Input: dimensioned drawing with shaded views. Units: mm. Origin: part minimum x, y, z. A direction names the side the tool comes from. Coordinates: 2 decimals unless noted, no trailing zeros. Loops run counter-clockwise (first coordinate to the right, second up) from the corner with the lowest first, then second, coordinate; pieces in that order, holes last. Notation, with made-up numbers: (11.5, 46) - (35.5, 46) arc R21 cw to (35.5, 63) - close; hole circle Ø8 at (62.25, 54.25). An arc over 180 degrees is marked (long way). Put each result on its own line as item: value. Start each with the question number.
1) Contact query for flat-ended pins moving along their axis: pin 1 Ø8 at (x, y) = (13.5, 17) entering from +Z; pin 2 Ø1 at (y, z) = (32, 7) entering from +X; pin 3 Ø6 at (x, y) = (47, 29.5) entering from +Z. Output: stop coordinate, or through.
2) Section B-B on z = 19.75. Output: boundary loops of the cut face in (x, y) (1 decimal).
3) Draft query along Y for the marked faces 3, 4 and 5. Return one class per face: +Y half, -Y half, draft (parallel to the pull), parting line (faces both ways), or undercut.
4) Section A-A on y = 19.5. Output: boundary loops of the cut face in (x, z) (1 decimal).
5) Material intervals for line 1 along Y through (x, z) = (23, 23); line 2 along X through (y, z) = (25.5, 16.25) (1 decimal); line 3 along X through (y, z) = (18.5, 4), sorted ascending. Write a range as from..to.
6) Section D-D on z = 7.5. Output: boundary loops of the cut face in (x, y) (1 decimal), and give its area (3 significant figures).
7) Reachability of the marked faces 1 and 2 from +Z, -Z, +X, -X, +Y, -Y: full face, straight path, thin tool, end or side. Return the list, or none.
8) Section C-C on x = 21.5. Output: boundary loops of the cut face in (y, z) (1 decimal).
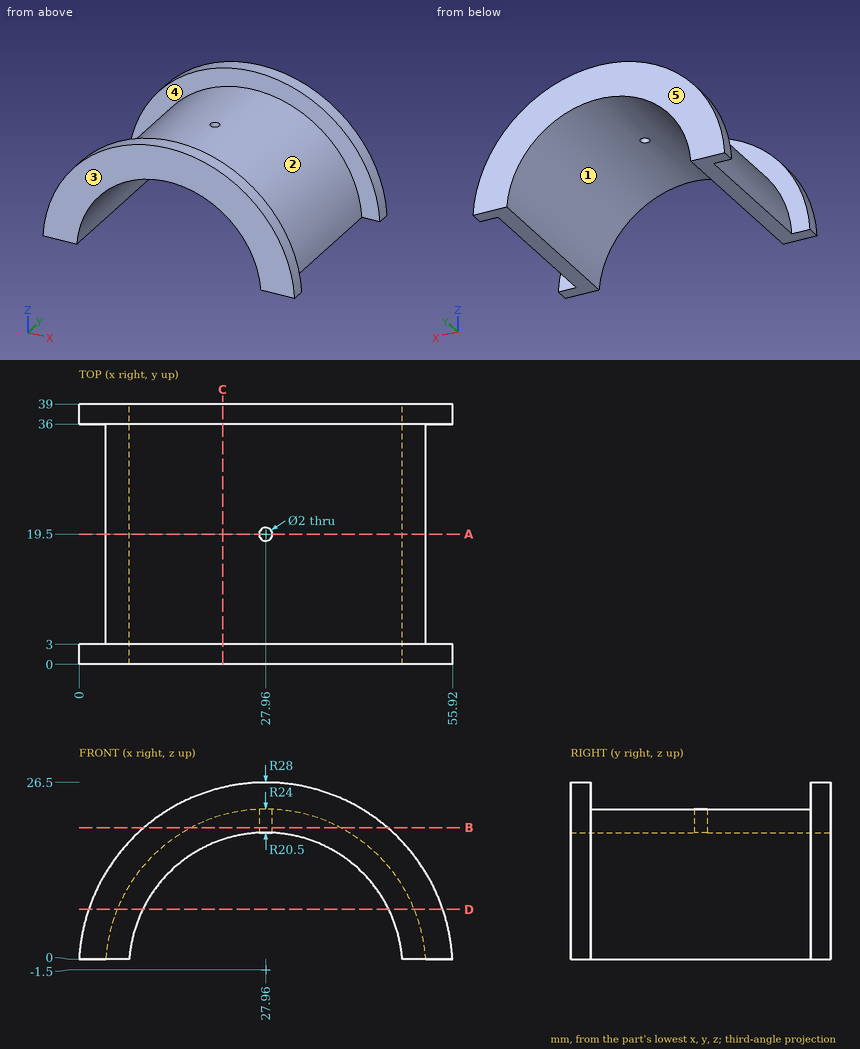
Answer block:
1. pin 1: stops at z = 20.1
1. pin 2: stops at x = 50.59
1. pin 3: stops at z = 16.35
2. outline: (9.7, 0) - (46.2, 0) - (46.2, 3) - (39.1, 3) - (39.1, 36) - (46.2, 36) - (46.2, 39) - (9.7, 39) - (9.7, 36) - (16.8, 36) - (16.8, 3) - (9.7, 3) - close; hole circle Ø2 at (28, 19.5)
3. face 3: -Y half
3. face 4: undercut
3. face 5: +Y half
4. outline: (4, 0) - (7.5, 0) arc R20.5 cw to (27, 19) - (27, 22.5) arc R24 ccw to start; (29, 19) arc R20.5 cw to (48.4, 0) - (51.9, 0) arc R24 ccw to (29, 22.5) - close
5. line 1: y = 0..3, 36..39
5. line 2: x = 11.8..17.7, 38.2..44.1
5. line 3: x = 4.6..8.21, 47.71..51.32
6. outline: (1.4, 0) - (9.5, 0) - (9.5, 39) - (1.4, 39) - (1.4, 36) - (5.7, 36) - (5.7, 3) - (1.4, 3) - close; (46.4, 0) - (54.5, 0) - (54.5, 3) - (50.2, 3) - (50.2, 36) - (54.5, 36) - (54.5, 39) - (46.4, 39) - close
6. area: 350 mm²
7. face 1: -Z, +Y, -Y
7. face 2: +Z
8. outline: (0, 18) - (39, 18) - (39, 25.7) - (36, 25.7) - (36, 21.6) - (3, 21.6) - (3, 25.7) - (0, 25.7) - close
